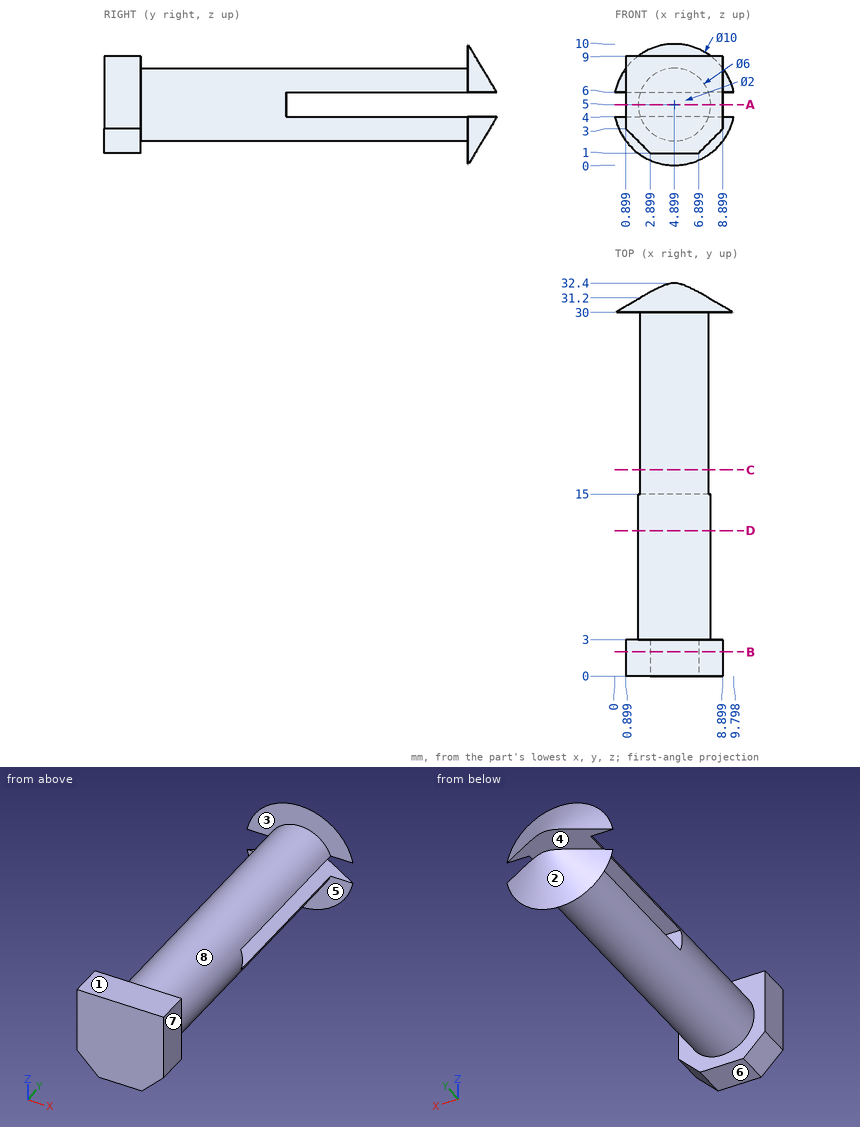
Print and shaded views of the part. All mm, measured from the part's lowest x, y and z. A direction names the side the tool comes from. Round coordinates to 2 decimals unless told otherwise and drop trailing zeros. Write each loop counter-clockwise with the first axis right and the second up, starting at its lowest first coordinate (ties: lowest second). Pieces come first, ordered by that corner, then holes. Notation, with made-up numbers: (64, -30) - (99, -30) arc R30 ccw to (99, 8) - close; hole circle Ø4 at (33.5, 62.25). An arc over 180 degrees is marked (long way). Write each question's results on one line, items separated by ' | '. Start each with the question number.
Item 1: Saw through at C-C (y = 17). Write the cut outline in (x, z).
Item 2: Wall check: L1, parallel to X at y = 12.5, z = 5; L2, parallel to Y at x = 2.25, z = 6.5; L3, parallel to Y at x = 8.25, z = 4.25. Give the ranges that are in metal, low to high. Write a range as [from, to].
Item 3: Saw through at B-B (y = 2). Write the cut outline in (x, z).
Item 4: Saw through at A-A (z = 5). Write the cut outline in (x, y).
Item 5: Drop flat-ended pins along their axis: P1, Ø1.6, axis at x = 5.5, z = 5.5, coming from the +Y side; P2, Ø2, axis at y = 18, z = 7.5, coming from the +X side; P3, Ø3, axis at x = 7, y = 23, coming from the -Z side; P4, Ø1, axis at y = 7, z = 2, coming from the +X side. Give the stop position or say it passes through.
Item 6: Mould opens along Y. For the marked faces 1, 2 and 3 say: pulls with the +Y half, pulls with the -Y half, needs draft (parallel to the pull), parting line crosses it, or undercut.
Item 7: Which spindle directions (+Z, -Z, +X, -X, +Y, -Y) get a long thin tool onto all of the face, cutting with end or side? Do the marked faces 4, 5, 6, 7 and 8. Say none if no direction does.
Item 8: Saw through at D-D (y = 12). Write the cut outline in (x, z), and give its area (3 significant figures).
Results are:
1) outline: (2.07, 4) arc R3 ccw to (7.73, 4) - close; (2.07, 6) - (7.73, 6) arc R3 ccw to start
2) L1: x = [1.9, 7.9] | L2: y = [0, 3], [30, 31.17] | L3: y = [0, 3]
3) outline: (0.9, 3) - (2.9, 1) - (6.9, 1) - (8.9, 3) - (8.9, 9) - (0.9, 9) - close
4) outline: (0.9, 0) - (8.9, 0) - (8.9, 3) - (7.9, 3) - (7.9, 15) - (1.9, 15) - (1.9, 3) - (0.9, 3) - close
5) P1: stops at y = 32.4 | P2: stops at x = 7.5 | P3: stops at z = 2.06 | P4: stops at x = 6.56
6) face 1: needs draft | face 2: pulls with the +Y half | face 3: undercut
7) face 4: +X, -X, +Y | face 5: -Z | face 6: -Z, +X, -X, -Y | face 7: +Z, -Z, +X, -Y | face 8: none
8) outline: circle Ø6 at (4.9, 5) | area: 28.3 mm²
